from build123d import *

# Parameters (mm, degrees)
SKETCH_1_R                = 20
EXTRUDE_1_DEPTH           = 60
EXTRUDE_1_TAPER           = 2
EXTRUDE_1_OTHER_WAY_DEPTH = 10


with BuildPart() as part:
    # Эскиз1 → Бобышка-Вытянуть1 (new body)
    with BuildSketch(Plane(origin=(0, 0, 0), x_dir=(1, 0, 0), z_dir=(0, 1, 0))):
        with Locations(Location((0, 0, 0), (0, 0, 270))):
            Circle(SKETCH_1_R)
    extrude(amount=EXTRUDE_1_DEPTH, taper=EXTRUDE_1_TAPER)

    # Эскиз1 → Бобышка-Вытянуть1 other way (add)
    with BuildSketch(Plane(origin=(0, 0, 0), x_dir=(1, 0, 0), z_dir=(0, 1, 0))):
        with Locations(Location((0, 0, 0), (0, 0, 270))):
            Circle(SKETCH_1_R)
    extrude(amount=-EXTRUDE_1_OTHER_WAY_DEPTH)

    # Эскиз3 → Вырез-Повернуть1 (revolve, cut)
    with BuildSketch(Plane.XY, mode=Mode.PRIVATE) as cut_revolve_1_sk:
        Polygon((-15.743928258, 60), (-17.001715566, 0), (-17.001715566, -7.030322503), (-9.901128706, -7.030322503), (0.031057723, -2.186071506), (-0.852425624, 60), align=None)
    revolve(cut_revolve_1_sk.sketch.rotate(Axis((0.031057723, -2.186071506, 0), (-0.014205660156622533, 0.9998990945187992, 0)), 180), axis=Axis((0.031057723, -2.186071506, 0), (-0.014205660156622533, 0.9998990945187992, 0)), mode=Mode.SUBTRACT)


solid = part.part
The listing builds one solid part. Answer for the finished solid, in the listing's coordinates (mm). A direction names the side the tool comes from. Give positions to 0.01 mm unless a question says otherwise; leave off trailing zeros.
Item 1: Determine the mould class of faces 3 (the cylindrical face through (-19.524, -4.93, -4.336)), 4 (the conical face through (16.31, -3.09, -5.12)), 5 (the flat face through (13.3, 60, 5.2)) for opening direction X: released by +X, released by -X, zero draft, split by the parting line, or undercut.
Item 2: Find the intervals of material crossed by line 1 along Z through (x, y) = (7, 14); line 2 along Z through (x, y) = (-12, 49.5); line 3 along X through (y, z) = (47, 5.5), in increasing order.
Item 3: Which of the six approach directions +Z, -Z, +X, -X, +Y, -Y give full straight-line access (tool end or side, diameter ignored) to faces 1 (the conical face through (-11.52, 30.42, -15.03)), 2 (the conical face through (-3.88, 29.76, 15.58))?
Item 4: Flat-ended cylindrical pins translate along their axes: P1, Ø5, axis at x = -7, z = -12.5, coming from the +Y side; P2, Ø12, axis at y = 44.5, z = -15.5, coming from the -X side; P3, Ø5, axis at y = 46.5, z = 12, coming from the -X side; P4, Ø10, axis at y = 18, z = -5.5, coming from the +X side. Find the tip coordinate at first contact, or state that the pin passes through.
Completed:
1. face 3: split by the parting line
1. face 4: undercut
1. face 5: zero draft
2. line 1: z = -18.21 to -14.87, 14.87 to 18.21
2. line 2: z = -13.78 to -10.26, 10.26 to 13.78
2. line 3: x = -17.52 to -15, 13.68 to 17.52
3. face 1: +Y
3. face 2: none
4. P1: stops at y = 60
4. P2: stops at x = -15.82
4. P3: stops at x = -15.73
4. P4: stops at x = 19.42
